```python
from build123d import *

# Parameters (mm, degrees)
SKETCH1_W           = 30
SKETCH1_H           = 30
BOSS_EXTRUDE1_DEPTH = 25
SKETCH2_W           = 10
SKETCH2_H           = 30
CUT_EXTRUDE1_DEPTH  = 5
SKETCH3_W           = 10
SKETCH3_H           = 30
CUT_EXTRUDE2_DEPTH  = 15
SKETCH4_W           = 10
SKETCH4_H           = 10
CUT_EXTRUDE3_DEPTH  = 15


with BuildPart() as part:
    # Sketch1 → Boss-Extrude1 (new body)
    with BuildSketch(Plane.XY):
        with Locations((15, 15)):
            Rectangle(SKETCH1_W, SKETCH1_H)
    extrude(amount=BOSS_EXTRUDE1_DEPTH)

    # Sketch2 → Cut-Extrude1 (cut)
    with BuildSketch(Plane.XY.offset(25)):
        with Locations((25, 15)):
            Rectangle(SKETCH2_W, SKETCH2_H)
    extrude(amount=-CUT_EXTRUDE1_DEPTH, mode=Mode.SUBTRACT)

    # Sketch3 → Cut-Extrude2 (cut)
    with BuildSketch(Plane.XY.offset(25)):
        with Locations((5, 15)):
            Rectangle(SKETCH3_W, SKETCH3_H)
    extrude(amount=-CUT_EXTRUDE2_DEPTH, mode=Mode.SUBTRACT)

    # Sketch4 → Cut-Extrude3 (cut)
    with BuildSketch(Plane(origin=(0, 30, 0), x_dir=(1, 0, 0), z_dir=(0, 1, 0))):
        with Locations((15, -20)):
            Rectangle(SKETCH4_W, SKETCH4_H)
    extrude(amount=-CUT_EXTRUDE3_DEPTH, mode=Mode.SUBTRACT)


solid = part.part
```
Geometry check sheet. Reference: the model listing, model coordinates, mm. A direction names the side the tool comes from. Round coordinates to 2 decimals unless told otherwise and drop trailing zeros. Order: outer loops, then holes, each group sorted by start corner. A loop starts at its lowest first (then second) coordinate and runs counter-clockwise, first axis right, second up. Notation, with made-up numbers: M 68,59.5 L 100,59.5 A28 ccw 100,83.5 Z; hole C 23,70.5 d10. An arc over 180 degrees is marked long. Answer as CSV lines item,"result".
1) Gauge pin test, flat ends, axial feed: pin 1 Ø1.5 at (y, z) = (20, 17.5) entering from -X; pin 2 Ø3 at (x, y) = (6, 14.5) entering from +Z; pin 3 Ø3 at (x, y) = (12.5, 25) entering from +Z. Record the tip position at first contact, or that the pin passes through.
Entries:
pin 1,"x = 20"
pin 2,"z = 10"
pin 3,"z = 15"
2) Sectioned sample at B-B on y = 16.25. Record the cut outline in (x, z), and give its area (3 significant figures).
Entries:
outline,"M 0,0 L 30,0 L 30,20 L 20,20 L 20,15 L 10,15 L 10,10 L 0,10 Z"
area,"450 mm2"
3) Tool access check on faces 1 (the face through (20, 7, 23)), 2 (the face through (5, 15, 10)), 3 (the face through (15, 15, 20)). Record the directions out of +Z, -Z, +X, -X, +Y, -Y that give a thin tool (end or side, any length) a straight path to the whole face; none if there is none.
Entries:
face 1,"+Z, +X, +Y, -Y"
face 2,"+Z, -X, +Y, -Y"
face 3,"+Z, -X, +Y"
4) Sectioned sample at D-D on y = 3. Record the cut outline in (x, z).
Entries:
outline,"M 0,0 L 30,0 L 30,20 L 20,20 L 20,25 L 10,25 L 10,10 L 0,10 Z"
5) Sectioned sample at A-A on z = 18. Record the cut outline in (x, y).
Entries:
outline,"M 10,0 L 30,0 L 30,30 L 20,30 L 20,15 L 10,15 Z"
6) Thickness scan on probe 1 along Z at (x, y) = (10.5, 26.5); probe 2 along Z at (x, y) = (9.5, 22.75); probe 3 along X at (y, z) = (28.75, 17). Record the ranges inside material, lowest first. Write a range as [from, to].
Entries:
probe 1,"[0, 15]"
probe 2,"[0, 10]"
probe 3,"[20, 30]"
7) Sectioned sample at C-C on x = 17.25. Record the cut outline in (y, z).
Entries:
outline,"M 0,0 L 30,0 L 30,15 L 15,15 L 15,25 L 0,25 Z"
